Part model, mm, in its own coordinate system. A direction names the side the tool comes from. Round coordinates to 2 decimals unless told otherwise and drop trailing zeros. Write each loop counter-clockwise with the first axis right and the second up, starting at its lowest first coordinate (ties: lowest second). Pieces come first, ordered by that corner, then holes. Notation, with made-up numbers: (21.5, 8.5) -> (77.5, 8.5) arc R32 cw to (77.5, 38.5) -> close; hole circle Ø3 at (19, 25.5). An arc over 180 degrees is marked (long way). Use CSV: the item, a comma, the result in double quotes. Start each with the question number.
(1) Probe line 1 (Y direction, x = 4.5, z = -21); line 2 (Z direction, x = 0.5, y = -5.5); line 3 (Z direction, x = 1.75, y = -5) (3 decimals). List the from-to ranges inside material, lowest first. Write a range as [from, to].
(2) Saw through at B-B (x = 1). Count the separate pieces of the cut face and the enclosed holes in it, plus the area to 3 significant figures.
(3) Saw through at C-C (z = -56). Give the cut face in (x, y).
(4) Saw through at D-D (y = -13). Give the cut face in (x, z).
(5) Which spindle directions (+Z, -Z, +X, -X, +Y, -Y) get a long thin tool onto all of the face, cutting with end or side? Do faces 1 (the cylindrical face through (3.13, -0.69, -46.9)), 2 (the flat face through (3, -13, -38.815)), 3 (the flat face through (3, 13, -38.815)). Say none if no direction does.
(6) Saw through at A-A (z = 0). Give the cut face in (x, y) (3 decimals), plus the area to 3 significant figures.
(7) Drop flat-ended pins along their axis: pin 1 (4 mm diameter, centred on y = 0, z = -50, fed in from +X); pin 2 (3 mm diameter, centred on x = 4, y = -14, fed in from +Z); pin 3 (1.9 mm diameter, centred on x = 2.5, z = -13, fed in from -Y). Give the stop position or say it passes through.
(8) Two-plate mould, pull along Z, no slides. Class faces 4 (the flat face through (3, 8, -10)), 5 (the flat face through (3, -14, -67.5)), 6 (the cylindrical face through (3.13, -0.69, 3.1)): released by +Z, released by -Z, zero draft, split by the parting line, or undercut.
Autodesk Inventor part; units mm, degrees
ref_plane "YZ Plane" through (0, 0, 0) normal (1, 0, 0) x (0, 1, 0)
ref_plane "XZ Plane" through (0, 0, 0) normal (0, 1, 0) x (-1, 0, 0)
ref_plane "XY Plane" through (0, 0, 0) normal (0, 0, 1) x (1, 0, 0)
sketch "Block1" plane through (0, 0, 0) normal (0, 0, 1) x (1, 0, 0)
  circle A0 centre (-34.5082, -40.3774) radius 0.55
  circle A1 centre (-31.5082, -40.3774) radius 0.55
  circle A2 centre (-28.5082, -40.3774) radius 0.55
  point P0 (-31.5082, -40.3774)
  dimension "d7" = 1.1
  dimension "d8" = 1.1
  dimension "d9" = 1.1
sketch "Sketch1" plane through (0, 0, 0) normal (1, 0, 0) x (0, 1, 0)
  circle A0 centre (0, 0) radius 3.175
  line L0 (8, 0) -> (8, -50)
  line L1 (-8, 0) -> (-8, -50)
  arc A1 (-8, -50) -> (8, -50) centre (0, -50) ccw
  circle A2 centre (0, -50) radius 3.175
  line L2 (0, -86.2) -> (0, 44.7) construction
  line L3 (8, 0) -> (-8, 0) construction
  line L4 (8, 0) -> (8, 18)
  line L5 (-8, 0) -> (-8, 18)
  arc A3 (8, 18) -> (-8, 18) centre (0, 18) ccw
  line L6 (-25.2, 0) -> (25.2, 0) construction
  line L7 (-8, -42.5) -> (-18, -42.5)
  line L8 (-18, -42.5) -> (-18, -67.5)
  line L9 (-18, -67.5) -> (-8, -67.5)
  line L10 (-8, -67.5) -> (-8, -42.5)
  line L11 (-8, -42.5) -> (17.0955, -42.5) construction
  line L12 (-8, -50) -> (-18, -50)
  line L13 (-18, -50) -> (-18, -38.8151)
  line L14 (-18, -38.8151) -> (-8, -38.8151)
  line L15 (-8, -38.8151) -> (-8, -50)
  line L16 (-8, -50) -> (-10.3039, -67.5)
  line L17 (-8, -50) -> (9.651, -50) construction
  line L18 (8, -42.5) -> (18, -42.5)
  line L19 (18, -42.5) -> (18, -67.5)
  line L20 (18, -67.5) -> (8, -67.5)
  line L21 (8, -67.5) -> (8, -42.5)
  line L22 (8, -50) -> (18, -50)
  line L23 (18, -50) -> (18, -38.8151)
  line L24 (18, -38.8151) -> (8, -38.8151)
  line L25 (8, -38.8151) -> (8, -50)
  line L26 (8, -50) -> (10.3039, -67.5)
  circle A4 centre (0, -12) radius 0.55
  circle A5 centre (0, -15) radius 0.55
  circle A6 centre (0, -18) radius 0.55
  circle A7 centre (0, 12) radius 0.55
  circle A8 centre (0, 15) radius 0.55
  circle A9 centre (0, 18) radius 0.55
  point P0 (0, 0)
  point P1 (-8, -25)
  dimension "d0" = 6.35
  dimension "d2" = 16
  dimension "d4" = 6.35
  dimension "d11" = 12
  dimension "d12" = 50
  dimension "d16" = 10
  dimension "d17" = 25
  dimension "d18" = 42.5
  dimension "d20" = 10
  dimension "d21" = 97.5
extrude "Extrusion1" add sketch "Sketch1" along normal blind 6.35 contours L0 A1 L1 L5 A3 L4 | L24 L23 L18 L0 | L18 L19 L22 L0 | L22 L19 L20 L26 | L12 L8 L7 L1 | L16 L9 L8 L12 | L1 L7 L13 L14
equation "\"d7\" = d9"
equation "\"d8\" = d9"
properties part number "Crank Skiba"
Answers:
1,line 1,"y = [-8, 8]"
1,line 2,"z = [-55.81, 23.81]"
1,line 3,"z = [-56.245, 24.245]"
2,separate pieces,"1"
2,enclosed holes,"8"
2,area,"1,750 mm²"
3,outline,"(0, -18) -> (6.35, -18) -> (6.35, -8.79) -> (0, -8.79) -> close; (0, -5.29) -> (6.35, -5.29) -> (6.35, 5.29) -> (0, 5.29) -> close; (0, 8.79) -> (6.35, 8.79) -> (6.35, 18) -> (0, 18) -> close"
4,outline,"(0, -67.5) -> (6.35, -67.5) -> (6.35, -38.82) -> (0, -38.82) -> close"
5,face 1,"+X, -X"
5,face 2,"+Z, +X, -X, -Y"
5,face 3,"+Z, +X, -X, +Y"
6,outline,"(0, -8) -> (6.35, -8) -> (6.35, -3.175) -> (0, -3.175) -> close; (0, 3.175) -> (6.35, 3.175) -> (6.35, 8) -> (0, 8) -> close"
6,area,"61.3 mm²"
7,pin 1,"passes through"
7,pin 2,"stops at z = -38.82"
7,pin 3,"stops at y = -8"
8,face 4,"zero draft"
8,face 5,"released by -Z"
8,face 6,"undercut"
